```python
from build123d import *

# Parameters (mm, degrees)
EXTRUDE_2_DEPTH = 3
SKETCH_1_5_W    = 100
SKETCH_1_5_H    = 80
SKETCH_1_5_R    = 1.5
EXTRUDE_3_DEPTH = 3


with BuildPart() as part:
    # 草图1 → 凸台-拉伸2 (new body)
    with BuildSketch(Plane.XY):
        with BuildLine():
            Line((-35.312957429, 30.171303214), (0, 1.920937271))
            Line((0, 1.920937271), (35.312957429, 30.171303214))
            ThreePointArc((35.312957429, 30.171303214), (37.421303214, 29.937042571), (37.187042571, 27.828696786))
            Line((37.187042571, 27.828696786), (2.401171589, 0))
            Line((2.401171589, 0), (37.187042571, -27.828696786))
            ThreePointArc((37.187042571, -27.828696786), (37.421303214, -29.937042571), (35.312957429, -30.171303214))
            Line((35.312957429, -30.171303214), (0, -1.920937271))
            Line((0, -1.920937271), (-35.312957429, -30.171303214))
            ThreePointArc((-35.312957429, -30.171303214), (-37.421303214, -29.937042571), (-37.187042571, -27.828696786))
            Line((-37.187042571, -27.828696786), (-2.401171589, 0))
            Line((-2.401171589, 0), (-37.187042571, 27.828696786))
            ThreePointArc((-37.187042571, 27.828696786), (-37.421303214, 29.937042571), (-35.312957429, 30.171303214))
        make_face()
    extrude(amount=EXTRUDE_2_DEPTH)

    # 草图1<5> → 凸台-拉伸3 (add)
    with BuildSketch(Plane.XY):
        Rectangle(SKETCH_1_5_W, SKETCH_1_5_H)
        with Locations((-43, -29)):
            Circle(SKETCH_1_5_R, mode=Mode.SUBTRACT)
        with BuildLine():
            ThreePointArc((-45, -10.5), (-47.560660172, -11.560660172), (-46.5, -9))
            ThreePointArc((-46.5, -9), (-45.439339828, -9.439339828), (-45, -10.5))
        make_face(mode=Mode.SUBTRACT)
        with Locations((43, -29)):
            Circle(SKETCH_1_5_R, mode=Mode.SUBTRACT)
        with Locations((43.5, -6.5)):
            Circle(SKETCH_1_5_R, mode=Mode.SUBTRACT)
        with BuildLine():
            ThreePointArc((-45, 10.5), (-45.439339828, 9.439339828), (-46.5, 9))
            ThreePointArc((-46.5, 9), (-47.560660172, 11.560660172), (-45, 10.5))
        make_face(mode=Mode.SUBTRACT)
        with Locations((-43, 29)):
            Circle(SKETCH_1_5_R, mode=Mode.SUBTRACT)
        with BuildLine():
            ThreePointArc((-37.187042571, 27.828696786), (-37.421303214, 29.937042571), (-35.312957429, 30.171303214))
            Line((-35.312957429, 30.171303214), (35.312957429, 30.171303214))
            ThreePointArc((35.312957429, 30.171303214), (37.421303214, 29.937042571), (37.187042571, 27.828696786))
            Line((37.187042571, 27.828696786), (37.187042571, -27.828696786))
            ThreePointArc((37.187042571, -27.828696786), (37.421303214, -29.937042571), (35.312957429, -30.171303214))
            Line((35.312957429, -30.171303214), (-35.312957429, -30.171303214))
            ThreePointArc((-35.312957429, -30.171303214), (-37.421303214, -29.937042571), (-37.187042571, -27.828696786))
            Line((-37.187042571, -27.828696786), (-37.187042571, 27.828696786))
        make_face(mode=Mode.SUBTRACT)
        with Locations((43, 29)):
            Circle(SKETCH_1_5_R, mode=Mode.SUBTRACT)
    extrude(amount=EXTRUDE_3_DEPTH)


solid = part.part
```
Work out the finished part from the listing and answer in its coordinate system (mm). A direction names the side the tool comes from. Coordinates: 2 decimals unless noted, no trailing zeros. Loops run counter-clockwise (first coordinate to the right, second up) from the corner with the lowest first, then second, coordinate; pieces in that order, holes last.
1) For a pull along X with two mould halves and no side action, classify faces 3 (the flat face through (50, -1, 1)), 4 (the flat face through (-1, 1, 0)), 5 (the cylindrical face through (41.89, 30.01, 1.48)) as +X half, -X half, draft (parallel to the pull), parting line (faces both ways), or undercut.
Results:
face 3: +X half
face 4: draft
face 5: undercut
2) Consider probe 1 along Y at (x, z) = (-46.5, 1.8); probe 2 along Y at (x, z) = (-43, 1.25); probe 3 along X at (y, z) = (16, 1.4). Determine where each line is inside the solid, lowest interval first.
Results:
probe 1: y = -40 to -12, -9 to 9, 12 to 40
probe 2: y = -40 to -30.5, -27.5 to 27.5, 30.5 to 40
probe 3: x = -50 to -37.19, -22.4 to -17.6, 17.6 to 22.4, 37.19 to 50
3) A flat-ended cylindrical pin translates along its axis: pin 1 (2.5 mm diameter, centred on x = 43, y = -29, fed in from -Z). Find the tip coordinate at first contact, or state that the pin passes through.
Results:
pin 1: passes through
4) For faces 1 (the flat face through (-17.9, 16.24, 1.48)), 2 (the flat face through (-1, 1, 3)), determine the directions among +Z, -Z, +X, -X, +Y, -Y from which every point of the face is accessible in a straight line to the end or side of a thin tool.
Results:
face 1: +Z, -Z
face 2: +Z, +X, -X, +Y, -Y
5) Section A-A (x = -43) is taken. Give the vertices of the cut face in (y, z).
Results:
outline: (-40, 0) - (-30.5, 0) - (-30.5, 3) - (-40, 3) - close; (-27.5, 0) - (27.5, 0) - (27.5, 3) - (-27.5, 3) - close; (30.5, 0) - (40, 0) - (40, 3) - (30.5, 3) - close
6) Section C-C (z = 1.75) is taken. Give the number of separate pieces and of enclosed holes in the cut face, plus the area to 3 significant figures.
Results:
separate pieces: 1
enclosed holes: 11
area: 4,020 mm2
7) Section D-D (x = 15) is taken. Give the vertices of the cut face in (y, z).
Results:
outline: (-40, 0) - (-30.17, 0) - (-30.17, 3) - (-40, 3) - close; (-13.92, 0) - (-10.08, 0) - (-10.08, 3) - (-13.92, 3) - close; (10.08, 0) - (13.92, 0) - (13.92, 3) - (10.08, 3) - close; (30.17, 0) - (40, 0) - (40, 3) - (30.17, 3) - close
8) Section B-B (y = -29) is taken. Give the vertices of the cut face in (x, z), plus the area to 3 significant figures.
Results:
outline: (-50, 0) - (-44.5, 0) - (-44.5, 3) - (-50, 3) - close; (-41.5, 0) - (-33.85, 0) - (-33.85, 3) - (-41.5, 3) - close; (33.85, 0) - (41.5, 0) - (41.5, 3) - (33.85, 3) - close; (44.5, 0) - (50, 0) - (50, 3) - (44.5, 3) - close
area: 78.9 mm2
